Input: part model. Units: mm. Frame: model coordinates. Face numbers are marked on the shaded views. A direction names the side the tool comes from. Give positions to 0.01 mm unless a question says otherwise; leave off trailing zeros. Loops run counter-clockwise (first coordinate to the right, second up) from the corner with the lowest first, then second, coordinate; pieces in that order, holes last. Notation, with made-up numbers: M -17.5,29.25 L -0.5,29.25 A35 ccw -0.5,68.25 Z; hole C -12,-16 d8. An arc over 180 degrees is marked long. One line per item, written item: value. Start each with the question number.
(1) Access query for the marked faces 5 and 6. Directions: +Z, -Z, +X, -X, +Y, -Y. A direction counts if a zero-diameter tool reaches every point of the face in a straight line with its end or side. Return the directions, or none.
(2) Section B-B on x = 20.5. Output: boundary loops of the cut face in (y, z), plus the area to 3 significant figures.
(3) Section C-C on x = 35. State how many separate pieces and enclosed holes the cut face has, plus the area to 3 significant figures.
(4) Section D-D on y = -67. Output: boundary loops of the cut face in (x, z), plus the area to 3 significant figures.
(5) Ray query, line 1 along X through (y, z) = (-36.5, -5.5); line 2 along X through (y, z) = (-61, 9.25); line 3 along Y through (x, z) = (36, 2.75). Return the intervals inside material, ascending. Write a range as from..to.
(6) Pin query (flat end, axial travel): P1, Ø12.5, axis at y = -38.5, z = -2.5, coming from the -X side; P2, Ø2, axis at x = 25.5, z = 9, coming from the +Y side; P3, Ø2.5, axis at y = -57.5, z = -2, coming from the -X side. Return the tip coordinate at first contact, or that it passes through.
(7) Pull-direction query (Y, two-part tool) for the marked faces 1, 2, 3 and 4; classes: released by +Y, released by -Y, zero draft, split by the parting line, or undercut.
(8) Section A-A on z = -6. Output: boundary loops of the cut face in (x, y), plus the area to 3 significant figures.
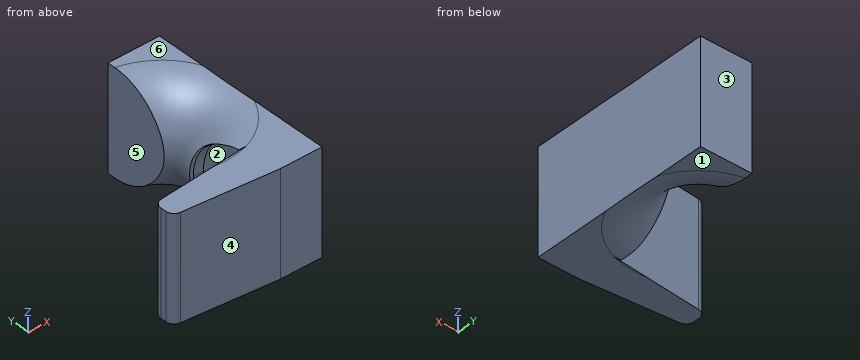
```python
from build123d import *

# Parameters (mm, degrees)
BOSS_EXTRUDE1_DEPTH = 12.5
BOSS_EXTRUDE2_DEPTH = 2.429285786
FILLET2_R           = 2


with BuildPart() as part:
    # Sketch2 → Boss-Extrude1 (new, symmetric)
    with BuildSketch(Plane.XY):
        Polygon((33.927983868, -28.997706932), (33.927983868, -52.497706932), (36.357269654, -52.497706932), (36.357269654, -64.539943653), (12.14546184, -66.65820236), (12.14546184, -71.65820236), (36.357269654, -73.776461068), (46.357269654, -73.776461068), (46.357269654, -28.997706932), align=None)
    extrude(amount=BOSS_EXTRUDE1_DEPTH, both=True)

    # Sketch4 → Boss-Extrude2 (add)
    with BuildSketch(Plane.ZY.offset(-36.357269654)):
        with BuildLine():
            Line((-12.5, -52.497706932), (-12.5, -64.539943653))
            Line((-12.5, -64.539943653), (-12.491615299, -64.539943653))
            ThreePointArc((-12.491615299, -64.539943653), (-8.675481514, -55.998483605), (0, -52.497706932))
            Line((0, -52.497706932), (-12.5, -52.497706932))
        make_face()
        with BuildLine():
            Line((12.5, -52.497706932), (0, -52.497706932))
            ThreePointArc((0, -52.497706932), (8.675481514, -55.998483605), (12.491615299, -64.539943653))
            Line((12.491615299, -64.539943653), (12.5, -64.539943653))
            Line((12.5, -64.539943653), (12.5, -52.497706932))
        make_face()
    extrude(amount=BOSS_EXTRUDE2_DEPTH)

    # Sketch3 → Cut-Revolve1 (revolve, cut)
    with BuildSketch(Plane.ZY.offset(-30.357269654)):
        with BuildLine():
            Line((-12.5, -47.997706932), (12.5, -47.997706932))
            Line((12.5, -47.997706932), (12.5, -30.497706932))
            ThreePointArc((12.5, -30.497706932), (0, -42.997706932), (-12.5, -30.497706932))
            Line((-12.5, -30.497706932), (-12.5, -47.997706932))
        make_face()
    revolve(axis=Axis((30.357269654, -47.997706932, -12.5), (0, 0, 1)), mode=Mode.SUBTRACT)

    # Fillet2
    fillet2_edges = [part.edges().sort_by_distance(p)[0] for p in [
        (12.14546184, -71.65820236, 0),
        (12.14546184, -66.65820236, 0),
    ]]
    fillet(fillet2_edges, radius=FILLET2_R)


solid = part.part
```
Output values:
1. face 5: +Z, -Z, -X, +Y
1. face 6: +Z, +X, -X, +Y, -Y
2. outline: M -72.39,-12.5 L -65.93,-12.5 L -65.93,12.5 L -72.39,12.5 Z
2. area: 162 mm²
3. separate pieces: 3
3. enclosed holes: 0
3. area: 592 mm²
4. outline: M 12.81,-12.5 L 46.36,-12.5 L 46.36,12.5 L 12.81,12.5 Z
4. area: 839 mm²
5. line 1: x = 33.93..46.36
5. line 2: x = 36.36..46.36
5. line 3: y = -73.75..-64.57, -52.8..-29
6. P1: stops at x = 33.93
6. P2: stops at y = -65.4
6. P3: stops at x = 36.36
7. face 1: zero draft
7. face 2: undercut
7. face 3: released by +Y
7. face 4: released by -Y
8. outline: M 12.15,-69.83 A2 ccw 13.97,-71.82 L 36.36,-73.78 L 46.36,-73.78 L 46.36,-29 L 33.93,-29 L 33.93,-42.53 A6.53 cw 33.93,-53.47 L 33.93,-54.03 L 36.36,-54.03 L 36.36,-64.54 L 13.97,-66.5 A2 ccw 12.15,-68.49 Z
8. area: 657 mm²
